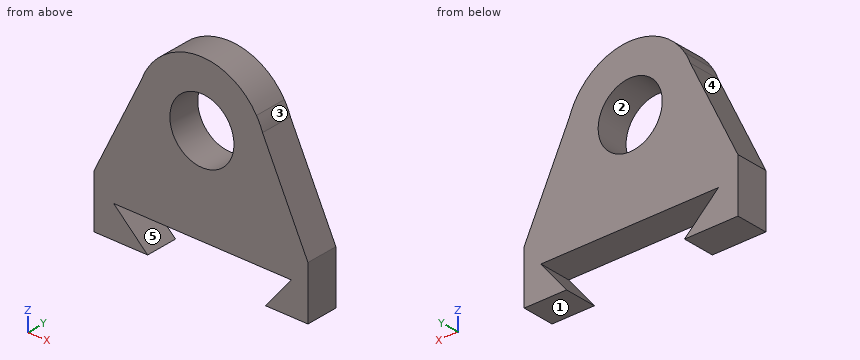
from build123d import *

# Parameters (mm, degrees)
F0_R     = 30
F1_DEPTH = 25
F2_DEPTH = 30


with BuildPart() as f1:
    # F0 (on Front) → F1 (new body)
    with BuildSketch(Plane.XZ):
        with BuildLine():
            Line((-56.185745, 83.036698), (-100.799982, -8.014716))
            Line((-100.799982, -8.014716), (99.200018, -8.014716))
            Line((99.200018, -8.014716), (56.705809, 81.592712))
            ThreePointArc((56.705809, 81.592712), (59.170721, 71.926398), (60, 61.985284))
            ThreePointArc((60, 61.985284), (-10.697086, 2.946548), (-56.185745, 83.036698))
        make_face()
        Polygon((99.200018, -8.014716), (-100.799982, -8.014716), (-100.799982, -58.014716), (-50.799982, -58.014716), (-82.59998, -28.014716), (83.600022, -28.014716), (59.600013, -58.014716), (99.200018, -58.014716), align=None)
        with BuildLine():
            Line((-51.065717, 93.48596), (-56.185745, 83.036698))
            ThreePointArc((-56.185745, 83.036698), (-10.697086, 2.946548), (60, 61.985284))
            ThreePointArc((60, 61.985284), (59.170721, 71.926398), (56.705809, 81.592712))
            Line((56.705809, 81.592712), (51.065717, 93.48596))
            ThreePointArc((51.065717, 93.48596), (0, 121.985284), (-51.065717, 93.48596))
        make_face()
        with Locations((0, 61.985284)):
            Circle(F0_R, mode=Mode.SUBTRACT)
        with BuildLine():
            ThreePointArc((-51.065717, 93.48596), (-53.879642, 88.385743), (-56.185745, 83.036698))
            Line((-56.185745, 83.036698), (-51.065717, 93.48596))
        make_face()
        with BuildLine():
            Line((51.065717, 93.48596), (56.705809, 81.592712))
            ThreePointArc((56.705809, 81.592712), (54.212893, 87.69447), (51.065717, 93.48596))
        make_face()
    extrude(amount=F1_DEPTH)

    # F0 (on Front) → F2 (join)
    with BuildSketch(Plane.XZ):
        with BuildLine():
            Line((-56.185745, 83.036698), (-100.799982, -8.014716))
            Line((-100.799982, -8.014716), (99.200018, -8.014716))
            Line((99.200018, -8.014716), (56.705809, 81.592712))
            ThreePointArc((56.705809, 81.592712), (59.170721, 71.926398), (60, 61.985284))
            ThreePointArc((60, 61.985284), (-10.697086, 2.946548), (-56.185745, 83.036698))
        make_face()
        Polygon((99.200018, -8.014716), (-100.799982, -8.014716), (-100.799982, -58.014716), (-50.799982, -58.014716), (-82.59998, -28.014716), (83.600022, -28.014716), (59.600013, -58.014716), (99.200018, -58.014716), align=None)
        with BuildLine():
            Line((-51.065717, 93.48596), (-56.185745, 83.036698))
            ThreePointArc((-56.185745, 83.036698), (-10.697086, 2.946548), (60, 61.985284))
            ThreePointArc((60, 61.985284), (59.170721, 71.926398), (56.705809, 81.592712))
            Line((56.705809, 81.592712), (51.065717, 93.48596))
            ThreePointArc((51.065717, 93.48596), (0, 121.985284), (-51.065717, 93.48596))
        make_face()
        with Locations((0, 61.985284)):
            Circle(F0_R, mode=Mode.SUBTRACT)
        with BuildLine():
            ThreePointArc((-51.065717, 93.48596), (-53.879642, 88.385743), (-56.185745, 83.036698))
            Line((-56.185745, 83.036698), (-51.065717, 93.48596))
        make_face()
        with BuildLine():
            Line((51.065717, 93.48596), (56.705809, 81.592712))
            ThreePointArc((56.705809, 81.592712), (54.212893, 87.69447), (51.065717, 93.48596))
        make_face()
    extrude(amount=F2_DEPTH)


solid = f1.part
Geometry check sheet. Reference: the model listing, model coordinates, mm. Face numbers are marked on the shaded views. A direction names the side the tool comes from. Round coordinates to 2 decimals unless told otherwise and drop trailing zeros. Loops run counter-clockwise (first coordinate to the right, second up) from the corner with the lowest first, then second, coordinate; pieces in that order, holes last. Notation, with made-up numbers: (82.25, -40) -> (97.25, -40) arc R4 ccw to (97.25, -33) -> close; hole circle Ø2 at (54.5, -3.5). An arc over 180 degrees is marked (long way). Answer as a JSON object with one key per item and string values. Group by question number.
Item 1: Cross-section at B-B, the plane z = -31. Record the cut outline in (x, y), plus the area to 3 significant figures.
Item 2: Set-up check for the marked faces 4 and 5: record each of +Z, -Z, +X, -X, +Y, -Y from which the full face is reachable in a straight line by a thin tool's end or side.
Item 3: Cross-section at D-D, the plane z = 20. Record the cut outline in (x, y), plus the area to 3 significant figures.
Item 4: Cross-section at A-A, the plane x = 0. Record the cut outline in (y, z).
Item 5: Release check for a two-part mould opening along Z. For the marked faces 1, 2 and 3 record: pulls with the +Z half, pulls with the -Z half, needs draft (parallel to the pull), parting line crosses it, or undercut.
Item 6: Cross-section at C-C, the plane y = -20.5. Record the cut outline in (x, z).
Item 7: Thickness scan on line 1 along Z through (x, y) = (0, -12.5); line 2 along X through (y, z) = (-20, -40.5); line 3 along X through (y, z) = (-10.25, 42.5). Record the ranges inside material, lowest first.
Item 8: Depth check by flat-ended pin: pin 1 Ø10 at (x, y) = (43.5, -20.5) entering from -Z; pin 2 Ø1.5 at (x, y) = (34, -6.5) entering from +Z; pin 3 Ø6 at (x, y) = (-39, -6.5) entering from +Z. Enter the tip coordinate at first touch or a pass-through.
Determined:
{
 "1": {"outline": "(-100.8, -30) -> (-79.44, -30) -> (-79.44, 0) -> (-100.8, 0) -> close; (81.21, -30) -> (99.2, -30) -> (99.2, 0) -> (81.21, 0) -> close", "area": "1,180 mm²"},
 "2": {"face 4": "+Z, -X, +Y, -Y", "face 5": "+Y, -Y"},
 "3": {"outline": "(-87.07, -30) -> (85.91, -30) -> (85.91, 0) -> (-87.07, 0) -> close", "area": "5,190 mm²"},
 "4": {"outline": "(-30, -28.01) -> (0, -28.01) -> (0, 31.99) -> (-30, 31.99) -> close; (-30, 91.99) -> (0, 91.99) -> (0, 121.99) -> (-30, 121.99) -> close"},
 "5": {"face 1": "pulls with the -Z half", "face 2": "undercut", "face 3": "pulls with the +Z half"},
 "6": {"outline": "(-100.8, -58.01) -> (-50.8, -58.01) -> (-82.6, -28.01) -> (83.6, -28.01) -> (59.6, -58.01) -> (99.2, -58.01) -> (99.2, -8.01) -> (56.71, 81.59) arc R60 ccw to (51.07, 93.49) arc R60 ccw to (-51.07, 93.49) arc R60 ccw to (-56.19, 83.04) -> (-100.8, -8.01) -> close; hole circle Ø60 at (0, 61.99)"},
 "7": {"line 1": "z = -28.01 to 31.99, 91.99 to 121.99", "line 2": "x = -100.8 to -69.37, 73.61 to 99.2", "line 3": "x = -76.05 to -22.81, 22.81 to 75.24"},
 "8": {"pin 1": "stops at z = -28.01", "pin 2": "stops at z = 111.93", "pin 3": "stops at z = 109.99"}
}
